Part print with two shaded views. Sizes in mm from the minimum x, y, z corner. A direction names the side the tool comes from. Give positions to 0.01 mm unless a question says otherwise; leave off trailing zeros. Loops run counter-clockwise (first coordinate to the right, second up) from the corner with the lowest first, then second, coordinate; pieces in that order, holes last. Notation, with made-up numbers: M -34.75,82 L -12.75,82 A18 cw -12.75,100 Z; hole C 10,1 d5. An arc over 180 degrees is marked long. Answer in a Markdown table with one row per item.
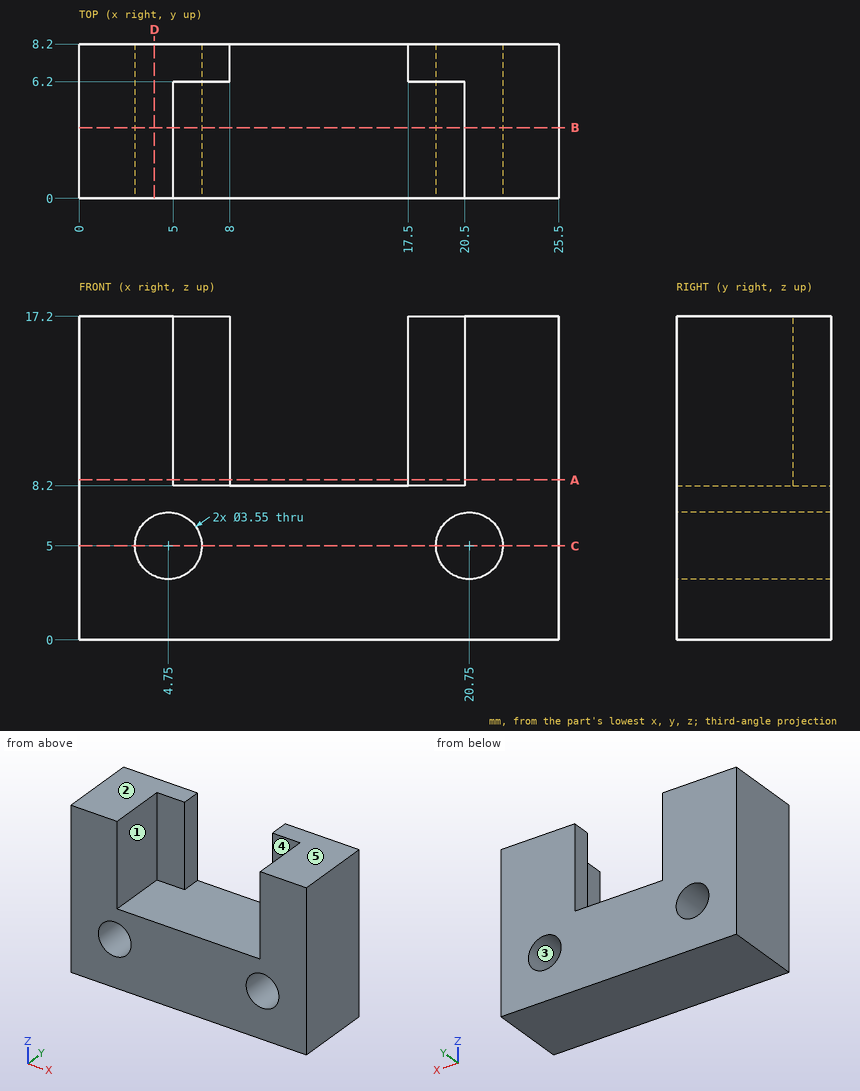
Q1. Saw through at C-C (z = 5). Give the cut face in (x, y) (3 decimals).
Reported:
| item | result |
|---|---|
| outline | M 0,0 L 2.975,0 L 2.975,8.2 L 0,8.2 Z; M 6.525,0 L 18.975,0 L 18.975,8.2 L 6.525,8.2 Z; M 22.525,0 L 25.5,0 L 25.5,8.2 L 22.525,8.2 Z |
Q2. Probe probe 1 along X at (y, z) = (4.75, 5) (3 decimals); probe 2 along Z at (x, y) = (20.75, 5.75) (3 decimals); probe 3 along X at (y, z) = (6, 15.25). List the from-to ranges inside material, lowest first.
Reported:
| item | result |
|---|---|
| probe 1 | 0 to 2.975, 6.525 to 18.975, 22.525 to 25.5 |
| probe 2 | 0 to 3.225, 6.775 to 17.2 |
| probe 3 | 0 to 5, 20.5 to 25.5 |
Q3. Saw through at D-D (x = 4). Give the cut face in (y, z), and give its area (3 significant figures).
Reported:
| item | result |
|---|---|
| outline | M 0,0 L 8.2,0 L 8.2,3.39 L 0,3.39 Z; M 0,6.61 L 8.2,6.61 L 8.2,17.2 L 0,17.2 Z |
| area | 115 mm² |
Q4. Saw through at A-A (z = 8.5). Give the cut face in (x, y), and give its area (3 significant figures).
Reported:
| item | result |
|---|---|
| outline | M 0,0 L 5,0 L 5,6.2 L 8,6.2 L 8,8.2 L 0,8.2 Z; M 17.5,6.2 L 20.5,6.2 L 20.5,0 L 25.5,0 L 25.5,8.2 L 17.5,8.2 Z |
| area | 94.0 mm² |
Q5. Mould opens along Z. For the marked faces 3, 4 and 5 say: released by +Z, released by -Z, zero draft, split by the parting line, or undercut.
Reported:
| item | result |
|---|---|
| face 3 | undercut |
| face 4 | zero draft |
| face 5 | released by +Z |
Q6. 3-axis set-ups, long thin cutter, end or side, ignore diameter. For the marked faces 1 and 2: which of +Z, -Z, +X, -X, +Y, -Y reach the whole face in a straight line?
Reported:
| item | result |
|---|---|
| face 1 | +Z, -Y |
| face 2 | +Z, +X, -X, +Y, -Y |
Q7. Saw through at B-B (y = 3.75). Give the cut face in (x, z) (3 decimals).
Reported:
| item | result |
|---|---|
| outline | M 0,0 L 25.5,0 L 25.5,17.2 L 20.5,17.2 L 20.5,8.2 L 5,8.2 L 5,17.2 L 0,17.2 Z; hole C 4.75,5 d3.55; hole C 20.75,5 d3.55 |
Q8. Drop flat-ended pins along their axis: pin 1 (2.5 mm diameter, centred on x = 12, y = 2.5, fed in from +Z); pin 2 (1.5 mm diameter, centred on x = 18.5, z = 11, fed in from -Y). Give the stop position or say it passes through.
Reported:
| item | result |
|---|---|
| pin 1 | z = 8.2 |
| pin 2 | y = 6.2 |
